Source: CAD feature listing. Evaluate the final solid. Frame: model axes, mm. A direction names the side the tool comes from. Round coordinates to 2 decimals unless told otherwise and drop trailing zeros. Loops run counter-clockwise (first coordinate to the right, second up) from the corner with the lowest first, then second, coordinate; pieces in that order, holes last.
Item 1: Access query for faces 1 (the flat face through (6, 15, -1.7)), 2 (the cylindrical face through (4.805, 26.487, -0.838)). Directions: +Z, -Z, +X, -X, +Y, -Y. A direction counts if a zero-diameter tool reaches every point of the face in a straight line with its end or side. Return the directions, or none.
Item 2: Ray query, L1, parallel to Y at x = 5, z = -0.95; L2, parallel to Y at x = 1.35, z = -15; L3, parallel to X at y = 28.5, z = -9. Return the intervals inside material, ascending.
Item 3: Section query B-B on z = -15. Return loops of the section in (x, y), then the cut area to 3 significant figures.
Item 4: First-contact query: P1, Ø5, axis at y = 21, z = -8, coming from the -X side; P2, Ø6, axis at x = 7, y = 12.5, coming from the -Z side. Flat tips, straight axial feed; report the tip coordinate or a pass-through.
Item 5: Section query C-C on x = 5. Return loops of the section in (y, z), then the cut area to 3 significant figures.
Item 6: Section query A-A on y = 5. Return loops of the section in (x, z).
Item 7: Pull-direction query (Z, two-part tool) for faces 3 (the cylindrical face through (0.84, 10.07, -16.5)), 4 (the flat face through (1, 0, -11)), 5 (the cylindrical face through (0.84, 21.01, -16.11)), 6 (the flat face through (1, 15, -25)); classes: released by +Z, released by -Z, zero draft, split by the parting line, or undercut.
Item 8: Section query D-D on x = 1.25. Return loops of the section in (y, z).
```python
from build123d import *

# Parameters (mm, degrees)
EXTRUDE_THIN1_DEPTH = 30
SKETCH10_R          = 1.5
CUT_EXTRUDE1_DEPTH  = 10
SKETCH11_R          = 1.5
CUT_EXTRUDE2_DEPTH  = 10
SKETCH12_W          = 15
SKETCH12_H          = 1.7
CUT_EXTRUDE3_DEPTH  = 40


with BuildPart() as part:
    # Sketch9 → Extrude-Thin1 (new body)
    with BuildSketch(Plane(origin=(0, 0, 0), x_dir=(1, 0, 0), z_dir=(0, 1, 0))):
        Polygon((0, 25), (0, 0), (25, 0), (25, 1.7), (1.7, 1.7), (1.7, 25), align=None)
    extrude(amount=EXTRUDE_THIN1_DEPTH)

    # Sketch10 → Cut-Extrude1 (cut)
    with BuildSketch(Plane.XY):
        with Locations((5, 25)):
            Circle(SKETCH10_R)
        with Locations((5, 5)):
            Circle(SKETCH10_R)
    extrude(amount=-CUT_EXTRUDE1_DEPTH, mode=Mode.SUBTRACT)

    # Sketch11 → Cut-Extrude2 (cut)
    with BuildSketch(Plane.ZY):
        with Locations((-15, 10)):
            Circle(SKETCH11_R)
        with Locations((-15, 20)):
            Circle(SKETCH11_R)
    extrude(amount=-CUT_EXTRUDE2_DEPTH, mode=Mode.SUBTRACT)

    # Sketch12 → Cut-Extrude3 (cut)
    with BuildSketch(Plane(origin=(0, 30, 0), x_dir=(1, 0, 0), z_dir=(0, 1, 0))):
        with Locations((17.5, 0.85)):
            Rectangle(SKETCH12_W, SKETCH12_H)
    extrude(amount=-CUT_EXTRUDE3_DEPTH, mode=Mode.SUBTRACT)


solid = part.part
```
Data:
1. face 1: -Z, +X, +Y, -Y
1. face 2: +Z, -Z
2. L1: y = 0 to 3.5, 6.5 to 23.5, 26.5 to 30
2. L2: y = 0 to 8.5, 11.5 to 18.5, 21.5 to 30
2. L3: x = 0 to 1.7
3. outline: (0, 0) - (1.7, 0) - (1.7, 8.5) - (0, 8.5) - close; (0, 11.5) - (1.7, 11.5) - (1.7, 18.5) - (0, 18.5) - close; (0, 21.5) - (1.7, 21.5) - (1.7, 30) - (0, 30) - close
3. area: 40.8 mm2
4. P1: stops at x = 0
4. P2: stops at z = -1.7
5. outline: (0, -1.7) - (3.5, -1.7) - (3.5, 0) - (0, 0) - close; (6.5, -1.7) - (23.5, -1.7) - (23.5, 0) - (6.5, 0) - close; (26.5, -1.7) - (30, -1.7) - (30, 0) - (26.5, 0) - close
5. area: 40.8 mm2
6. outline: (0, -25) - (1.7, -25) - (1.7, -1.7) - (3.5, -1.7) - (3.5, 0) - (0, 0) - close; (6.5, -1.7) - (10, -1.7) - (10, 0) - (6.5, 0) - close
7. face 3: undercut
7. face 4: zero draft
7. face 5: undercut
7. face 6: released by -Z
8. outline: (0, -25) - (30, -25) - (30, 0) - (0, 0) - close; hole circle Ø3 at (10, -15); hole circle Ø3 at (20, -15)
